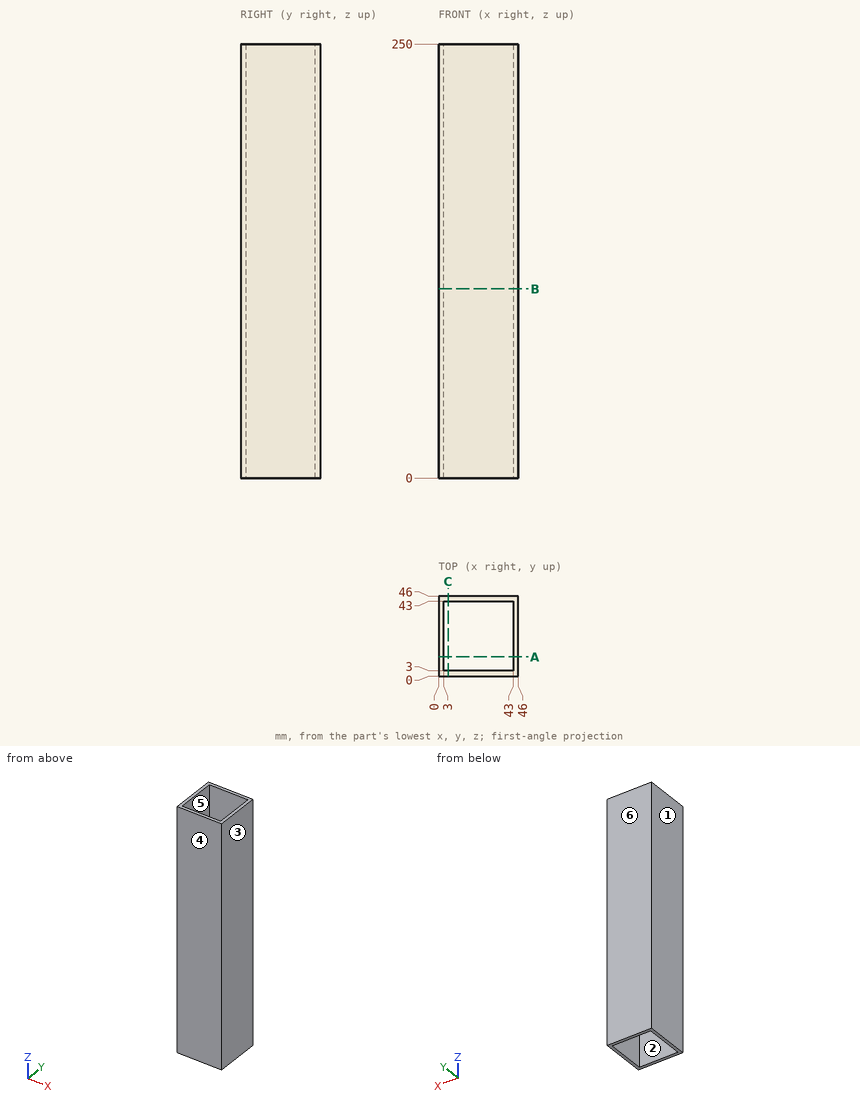
Geometry: see drawing. Coordinates: mm, zero at the bounding-box minimum. A direction names the side the tool comes from. Coordinates: 2 decimals unless noted, no trailing zeros. Order: outer loops, then holes, each group sorted by start corner. A loop starts at its lowest first (then second) coordinate and runs counter-clockwise, first axis right, second up. Notation, with made-up numbers: M 84.5,15.5 L 100.5,15.5 A23 cw 100.5,33.5 Z; hole C 35,-14 d11. An arc over 180 degrees is marked long. Answer as CSV lines item,"result".
1. Section A-A (y = 11). Return the cut outline in (x, z), then the cut area to 3 significant figures.
Reported:
outline,"M 0,0 L 3,0 L 3,250 L 0,250 Z; M 43,0 L 46,0 L 46,250 L 43,250 Z"
area,"1,500 mm2"
2. Access query for the marked faces 5 and 6. Directions: +Z, -Z, +X, -X, +Y, -Y. A direction counts if a zero-diameter tool reaches every point of the face in a straight line with its end or side. Return the directions, or none.
Reported:
face 5,"+Z, -Z"
face 6,"+Z, -Z, +X, -X, +Y"
3. Material intervals for line 1 (X direction, y = 30, z = 167), sorted ascending. Write a range as from..to.
Reported:
line 1,"0..3, 43..46"
4. Pull-direction query (X, two-part tool) for the marked faces 1, 2, 3 and 4; classes: released by +X, released by -X, zero draft, split by the parting line, or undercut.
Reported:
face 1,"released by -X"
face 2,"undercut"
face 3,"released by +X"
face 4,"zero draft"
5. Section B-B (z = 109). Return the cut outline in (x, y), then the cut area to 3 significant figures.
Reported:
outline,"M 0,0 L 46,0 L 46,46 L 0,46 Z; hole M 3,3 L 43,3 L 43,43 L 3,43 Z"
area,"516 mm2"
